Autodesk Fusion 360 part; units mm, degrees
sketch "Sketch1" plane through (0, 0, 0) normal (0, 1, 0) x (1, 0, 0)
  line L0 (-15, -9) -> (15, -9)
  line L1 (15, -9) -> (15, 9)
  line L2 (15, 9) -> (-15, 9)
  line L3 (-15, 9) -> (-15, -9)
  line L4 (-15, -9) -> (15, 9) construction
  line L5 (15, -9) -> (-15, 9) construction
  circle A0 centre (12.8, 0) radius 1.1
  circle A1 centre (-12.8, 0) radius 1.1
  dimension "d1" = 30
  dimension "d2" = 18
  dimension "d3" = 2.2
  dimension "d4" = 2.2
  dimension "d5" = 2.2
  dimension "d6" = 2.2
extrude "Extrude1" add sketch "Sketch1" along normal blind 1.6
Verification items for the finished model (mm, model axes). Round coordinates to 2 decimals unless told otherwise and drop trailing zeros. Loops run counter-clockwise (first coordinate to the right, second up) from the corner with the lowest first, then second, coordinate; pieces in that order, holes last. Notation, with made-up numbers: (64, -18.5) - (112, -18.5) arc R18 ccw to (112, 0.5) - close; hole circle Ø7 at (-35.75, 19). An arc over 180 degrees is marked (long way). Answer in a Markdown table with one row per item. Add a question column.
Q1. Release check for a two-part mould opening along X. For faces 1 (the face through (13.816, 0.789, -0.421)), 2 (the face through (0, 0, 0)), 3 (the face through (15, 1, 0)) record: pulls with the +X half, pulls with the -X half, needs draft (parallel to the pull), parting line crosses it, or undercut.
Q2. Section check B-B on x = 12.8. Enter the section's corners in (y, z).
Q3. Section check A-A on z = 0. Enter the section's corners in (x, y), plus the area to 3 significant figures.
Q4. Gauge pin test, flat ends, axial feed: pin 1 (1 mm diameter, centred on x = 8, z = 2.5, fed in from -Y); pin 2 (1.8 mm diameter, centred on x = 12.8, z = 0, fed in from -Y). Record the tip position at first contact, or that the pin passes through.
Q5. Material ranges on line 1 (X direction, y = 0.4, z = 0); line 2 (Z direction, x = 12.8, y = 1.05); line 3 (X direction, y = 0.55, z = -0.75), recorded low to high.
Found:
| question | item | result |
|---|---|---|
| 1 | face 1 | undercut |
| 1 | face 2 | needs draft |
| 1 | face 3 | pulls with the +X half |
| 2 | outline | (0, -9) - (1.6, -9) - (1.6, -1.1) - (0, -1.1) - close; (0, 1.1) - (1.6, 1.1) - (1.6, 9) - (0, 9) - close |
| 3 | outline | (-15, 0) - (-13.9, 0) - (-13.9, 1.6) - (-15, 1.6) - close; (-11.7, 0) - (11.7, 0) - (11.7, 1.6) - (-11.7, 1.6) - close; (13.9, 0) - (15, 0) - (15, 1.6) - (13.9, 1.6) - close |
| 3 | area | 41.0 mm² |
| 4 | pin 1 | stops at y = 0 |
| 4 | pin 2 | passes through |
| 5 | line 1 | x = -15 to -13.9, -11.7 to 11.7, 13.9 to 15 |
| 5 | line 2 | z = -9 to -1.1, 1.1 to 9 |
| 5 | line 3 | x = -15 to -13.6, -12 to 12, 13.6 to 15 |
